```python
from build123d import *

# Parameters (mm, degrees)
SKETCH1_W           = 10
SKETCH1_H           = 80
BOSS_EXTRUDE1_DEPTH = 10
SHELL1_T            = -1
FILLET1_R           = 0.75
SKETCH2_W           = 8.5
SKETCH2_H           = 20
BOSS_EXTRUDE2_DEPTH = 1
SKETCH3_W           = 0.75
SKETCH3_H           = 20
BOSS_EXTRUDE3_DEPTH = 30
CUT_EXTRUDE1_DEPTH  = 35
SKETCH5_R           = 2
CUT_EXTRUDE2_DEPTH  = 35
FILLET2_R           = 0.75
SKETCH6_R           = 2
BOSS_EXTRUDE4_DEPTH = 10


with BuildPart() as part:
    # Sketch1 → Boss-Extrude1 (new body)
    with BuildSketch(Plane.XY):
        Rectangle(SKETCH1_W, SKETCH1_H)
    extrude(amount=BOSS_EXTRUDE1_DEPTH)

    # Shell1
    shell1_openings = [part.faces().sort_by_distance(p)[0] for p in [
        (0, -40, 5),
        (0, 40, 5),
    ]]
    offset(amount=SHELL1_T, openings=shell1_openings, kind=Kind.INTERSECTION)

    # Fillet1
    fillet1_edges = [part.edges().sort_by_distance(p)[0] for p in [
        (-5, 0, 10),
        (5, 0, 10),
        (-5, 0, 0),
        (5, 0, 0),
    ]]
    fillet(fillet1_edges, radius=FILLET1_R)

    # Sketch2 → Boss-Extrude2 (add)
    with BuildSketch(Plane(origin=(5, 0, 0), x_dir=(0, 0, -1), z_dir=(1, 0, 0))):
        with Locations((-5, 15)):
            Rectangle(SKETCH2_W, SKETCH2_H)
    extrude(amount=BOSS_EXTRUDE2_DEPTH)

    # Sketch3 → Boss-Extrude3 (add)
    with BuildSketch(Plane(origin=(5, 0, 0), x_dir=(0, 0, -1), z_dir=(1, 0, 0))):
        with Locations((-9.625, 15)):
            Rectangle(SKETCH3_W, SKETCH3_H)
        with Locations((-0.375, 15)):
            Rectangle(SKETCH3_W, SKETCH3_H)
    extrude(amount=BOSS_EXTRUDE3_DEPTH)

    # Sketch4 → Cut-Extrude1 (cut)
    with BuildSketch(Plane.XY.offset(10)):
        Polygon((22, 5), (35, 5), (35, 25), (22, 25), (27.773502692, 15), align=None)
    extrude(amount=-CUT_EXTRUDE1_DEPTH, mode=Mode.SUBTRACT)

    # Sketch5 → Cut-Extrude2 (cut)
    with BuildSketch(Plane.XY.offset(10)):
        with Locations((0, 25)):
            Circle(SKETCH5_R)
        with Locations((0, -35)):
            Circle(SKETCH5_R)
        Polygon((-5, -35.5), (-0.5, -40), (-5, -40), align=None)
    extrude(amount=-CUT_EXTRUDE2_DEPTH, mode=Mode.SUBTRACT)

    # Fillet2
    fillet2_edges = [part.edges().sort_by_distance(p)[0] for p in [
        (1.875, -40, 0),
        (1.875, -40, 10),
        (-0.5, -40, 9.5),
        (-0.5, -40, 0.5),
        (5, -40, 5),
        (4.780330086, -40, 0.219669914),
        (4.780330086, -40, 9.780330086),
    ]]
    fillet(fillet2_edges, radius=FILLET2_R)

    # Sketch6 → Boss-Extrude4 (add)
    with BuildSketch(Plane.XY.offset(10)):
        with Locations((20, 15)):
            Circle(SKETCH6_R)
    extrude(amount=-BOSS_EXTRUDE4_DEPTH)


solid = part.part
```
Can you work these out from the model? Positions are in its coordinate system, mm. A direction names the side the tool comes from. Give positions to 0.01 mm unless a question says otherwise; leave off trailing zeros. Loops run counter-clockwise (first coordinate to the right, second up) from the corner with the lowest first, then second, coordinate; pieces in that order, holes last. Notation, with made-up numbers: M 40,-18 L 46,-18 A16 ccw 46,-5 Z; hole C -12.75,-32.5 d4. An arc over 180 degrees is marked long. Use one line per item in the form item = value. Start each with the question number.
(1) Thinking about a two-plate mould opening in Y: for faces 1 (the cylindrical face through (-0.434, -36.952, 9.507)), 2 (the cylindrical face through (-0.434, -36.952, 0.507)), 3 (the flat face through (-0.1, 40, 9.4)), 4 (the flat face through (5, 32, 5)), which applies, released by +Y, released by -Y, zero draft, split by the parting line, or undercut?
(2) I want a section at D-D, the plane x = 20. Write out the boundary of the cut face in (y, z).
(3) I want a section at A-A, the plane z = 2.25. Write out the boundary of the cut face in (x, y).
(4) On a 3-axis mill with a long thin cutter (end or side, diameter ignored), from which of +Z, -Z, +X, -X, +Y, -Y can I reach the whole of each face in a straight line? I mean faces 5 (the flat face through (10.9, 5, 9.5)), 6 (the flat face through (4, -1, 5)), 7 (the cylindrical face through (20, 17, 5)), 8 (the flat face through (10.9, 25, 9.5)). Say none if no direction works.
(5) I want a section at B-B, the plane y = -25. Write out the boundary of the cut face in (x, z).
(6) I'm going to push flat-ended pins straight in: P1, Ø9, axis at x = 0.5, y = -5.5, coming from the -Z side; P2, Ø4, axis at y = -24.5, z = 6.5, coming from the +X side; P3, Ø3.5, axis at x = 0, y = 25, coming from the +Z side; P4, Ø6, axis at x = 18.5, z = 8, coming from the +Y side. Where does each tip first touch, or does it pass through?
(7) Please list where these lines run through material, in increasing order: line 1 (Y direction, x = 0, z = 0.75); line 2 (X direction, y = -4, z = 5); line 3 (Z direction, x = 3, y = -34.5).
(8) I want a section at C-C, the plane x = 16.5. Write out the boundary of the cut face in (y, z).
Worked out:
q1.face_1 = undercut
q1.face_2 = undercut
q1.face_3 = released by +Y
q1.face_4 = zero draft
q2.outline = M 5,0 L 25,0 L 25,0.75 L 17,0.75 L 17,9.25 L 25,9.25 L 25,10 L 5,10 L 5,9.25 L 13,9.25 L 13,0.75 L 5,0.75 Z
q3.outline = M -5,-35.5 L -4,-36.5 L -4,40 L -5,40 Z; M 4,-40 L 4.25,-40 A0.75 ccw 5,-39.25 L 5,5 L 6,5 L 6,25 L 5,25 L 5,40 L 4,40 Z; C 20,15 d4
q4.face_5 = +Z, -Z, +X, -Y
q4.face_6 = +Y, -Y
q4.face_7 = none
q4.face_8 = +Z, -Z, +X, +Y
q5.outline = M -5,0.75 A0.75 ccw -4.25,0 L 4.25,0 A0.75 ccw 5,0.75 L 5,9.25 A0.75 ccw 4.25,10 L -4.25,10 A0.75 ccw -5,9.25 Z; hole M -4,1 L 4,1 L 4,9 L -4,9 Z
q6.P1 = 0
q6.P2 = 5
q6.P3 = through
q6.P4 = 25
q7.line_1 = -40 to -37, -33 to 23, 27 to 40
q7.line_2 = -5 to -4, 4 to 5
q7.line_3 = 0 to 1, 9 to 10
q8.outline = M 5,0 L 25,0 L 25,0.75 L 5,0.75 Z; M 5,9.25 L 25,9.25 L 25,10 L 5,10 Z
